For this review, take the finished solid that the model builds, in its own axes (mm). A direction names the side the tool comes from. Round coordinates to 2 decimals unless told otherwise and drop trailing zeros. Loops run counter-clockwise (first coordinate to the right, second up) from the corner with the lowest first, then second, coordinate; pieces in that order, holes last.
1) Take a section at B-B (x = 0). Give the number of separate pieces and of enclosed holes in the cut face, then the cut area to 3 significant figures.
2) Tool access review of faces 4 (the cylindrical face through (-0.632, 1.68, -9.476)), 5 (the cylindrical face through (-6.834, 5.698, -1.517)): name each direction out of +Z, -Z, +X, -X, +Y, -Y from which nothing blocks a thin tool from reaching the whole face with its end or side.
3) Insertion check: pin 1 (4 mm diameter, centred on x = 0, z = 11, fed in from +Y); pin 2 (5.5 mm diameter, centred on x = 0, z = -11, fed in from -Y); pin 3 (7 mm diameter, centred on x = 0, z = 0, fed in from +Y); pin 4 (1 mm diameter, centred on y = 1.5, z = -6.5, fed in from -X). Each pin has a flat end and moves straight along its axis. Give the tip position at first contact, or say it passes through.
4) Mouldability with a two-part tool opening along Z and no side actions: class faces 1 (the cylindrical face through (-3.905, 4.937, 0.867)), 2 (the cylindrical face through (0.66, 1.24, -14.985)), 3 (the flat face through (3.4, 0, -3.4)) as pulls with the +Z half, pulls with the -Z half, needs draft (parallel to the pull), parting line crosses it, or undercut.
5) Take a section at C-C (y = 6). State the section outline as (x, z) points.
6) Wall thickness on L1, parallel to X at y = 3.5, z = 0; L2, parallel to Y at x = -6.75, z = 4.5; L3, parallel to X at y = 4.5, z = -1.5: over which ranges is each line inside the solid? List them lowest first.
7) Take a section at A-A (z = 0). State the section outline as (x, y) points.
```python
from build123d import *

# Parameters (mm, degrees)
SKETCH_1_R                   = 15
EXTRUDE_1_DEPTH              = 2
SKETCH_2_R                   = 7
EXTRUDE_2_DEPTH              = 8
F_8_0MM_1_D                  = 8
HOLE_WIZARD_M6_1_D           = 3.3
HOLE_WIZARD_M6_1_CSINK_D     = 6
HOLE_WIZARD_M6_1_CSINK_ANGLE = 90
CHAMFER_1_SIZE               = 0.5


with BuildPart() as part:
    # 草图1 → 凸台-拉伸1 (new body)
    with BuildSketch(Plane(origin=(0, 0, 0), x_dir=(1, 0, 0), z_dir=(0, 1, 0))):
        with Locations(Location((0, 0, 0), (0, 0, 270))):
            Circle(SKETCH_1_R)
    extrude(amount=EXTRUDE_1_DEPTH)

    # 草图2 → 凸台-拉伸2 (add)
    with BuildSketch(Plane(origin=(0, 2, 0), x_dir=(1, 0, 0), z_dir=(0, 1, 0))):
        with Locations(Location((0, 0, 0), (0, 0, 270))):
            Circle(SKETCH_2_R)
    extrude(amount=EXTRUDE_2_DEPTH)

    # Ø8.0mm 暗销孔1 (through all)
    with Locations(Plane.ZX.offset(10)):
        with Locations((0, 0)):
            Hole(F_8_0MM_1_D / 2)

    # M6 内六角花形半沉头螺钉的锥形沉头孔1 (through all)
    with Locations(Plane(origin=(0, 0, -11), x_dir=(0, 0, -1), z_dir=(0, -1, 0))):
        with Locations((0, 0)):
            hole_wizard_m6_1 = CounterSinkHole(HOLE_WIZARD_M6_1_D / 2, HOLE_WIZARD_M6_1_CSINK_D / 2, counter_sink_angle=HOLE_WIZARD_M6_1_CSINK_ANGLE)

    # 镜向1: M6 内六角花形半沉头螺钉的锥形沉头孔1 across plane
    add(hole_wizard_m6_1.mirror(Plane.XY), mode=Mode.SUBTRACT)

    # 倒角1
    chamfer_1_edges = [part.edges().sort_by_distance(p)[0] for p in [
        (0, 10, 4),
        (0, 0, 4),
        (0, 0, -15),
        (0, 10, -7),
    ]]
    chamfer(chamfer_1_edges, length=CHAMFER_1_SIZE)


solid = part.part
```
Response:
1. separate pieces: 4
1. enclosed holes: 0
1. area: 74.2 mm2
2. face 4: +Y, -Y
2. face 5: +Y
3. pin 1: stops at y = 2
3. pin 2: stops at y = 0.25
3. pin 3: passes through
3. pin 4: stops at x = -13.75
4. face 1: undercut
4. face 2: parting line crosses it
4. face 3: needs draft
5. outline: circle Ø14 at (0, 0); hole circle Ø8 at (0, 0)
6. L1: x = -7 to -4, 4 to 7
6. L2: y = 0 to 2
6. L3: x = -6.84 to -3.71, 3.71 to 6.84
7. outline: (-15, 0.5) - (-14.5, 0) - (-4.5, 0) - (-4, 0.5) - (-4, 9.5) - (-4.5, 10) - (-6.5, 10) - (-7, 9.5) - (-7, 2) - (-15, 2) - close; (4, 0.5) - (4.5, 0) - (14.5, 0) - (15, 0.5) - (15, 2) - (7, 2) - (7, 9.5) - (6.5, 10) - (4.5, 10) - (4, 9.5) - close
